Geometry: final body of the model. Coordinates: model frame, mm. A direction names the side the tool comes from. Give positions to 0.01 mm unless a question says otherwise; leave off trailing zeros. Write each loop counter-clockwise with the first axis right and the second up, starting at its lowest first coordinate (ties: lowest second). Pieces come first, ordered by that corner, then holes.
```python
from build123d import *

# Parameters (mm, degrees)
F1_DEPTH = 5
F2_R     = 1.669174
F2_R_2   = 1.66634
F3_DEPTH = 40.001
F4_R     = 1.5
F5_DEPTH = 4.001


with BuildPart() as f1:
    # F0 (on Right) → F1 (new body)
    with BuildSketch(Plane.YZ):
        Polygon((16, -8.883437), (0, -8.883437), (-16, -8.883437), (-16, 29.116563), (-20, 29.116563), (-20, -12.883437), (0, -12.883437), (20, -12.883437), (20, 29.116563), (16, 29.116563), align=None)
    extrude(amount=F1_DEPTH)

    # F2 (on face) → F3 (cut, through all)
    with BuildSketch(Plane.XZ.offset(20)):
        with Locations((2.5, 17.616563)):
            Circle(F2_R)
        with Locations((2.5, 2.616563)):
            Circle(F2_R_2)
    extrude(amount=-F3_DEPTH, mode=Mode.SUBTRACT)

    # F4 (on face) → F5 (cut, through all)
    with BuildSketch(Plane.XY.offset(-8.883437)):
        with Locations((2.5, -8)):
            Circle(F4_R)
        with Locations((2.5, 8)):
            Circle(F4_R)
    extrude(amount=-F5_DEPTH, mode=Mode.SUBTRACT)


solid = f1.part
```
Item 1: Section D-D, the plane z = 17. Return the cut outline in (x, y), plus the area to 3 significant figures.
Found:
outline: (0, -20) - (0.95, -20) - (0.95, -16) - (0, -16) - close; (0, 16) - (0.95, 16) - (0.95, 20) - (0, 20) - close; (4.05, -20) - (5, -20) - (5, -16) - (4.05, -16) - close; (4.05, 16) - (5, 16) - (5, 20) - (4.05, 20) - close
area: 15.2 mm2
Item 2: Pull-direction query (X, two-part tool) for faces 1 (the face through (0, 1, -10)), 2 (the face through (2, 0, -8.883)), 3 (the face through (5, 1, -10)), 4 (the face through (0.832, -18.028, 17.69)); classes: +X half, -X half, draft (parallel to the pull), parting line (faces both ways), or undercut.
Found:
face 1: -X half
face 2: draft
face 3: +X half
face 4: undercut
Item 3: Section C-C, the plane z = -4.5. Return the cut outline in (x, y).
Found:
outline: (0, -20) - (5, -20) - (5, -16) - (0, -16) - close; (0, 16) - (5, 16) - (5, 20) - (0, 20) - close
Item 4: Section B-B, the plane x = 2.5. State how many separate pieces and enclosed holes the cut face has, plus the area to 3 significant figures.
Found:
separate pieces: 7
enclosed holes: 0
area: 387 mm2
Item 5: Line query: L1, parallel to Z at x = 2.5, y = 17.4; L2, parallel to Y at x = 2.5, z = -12.05; L3, parallel to Y at x = 3.75, z = -7. Output: solid intervals per line, ascending.
Found:
L1: z = -12.88 to 0.95, 4.28 to 15.95, 19.29 to 29.12
L2: y = -20 to -9.5, -6.5 to 6.5, 9.5 to 20
L3: y = -20 to -16, 16 to 20
Item 6: Section A-A, the plane y = 8. Return the cut outline in (x, z), plus the area to 3 significant figures.
Found:
outline: (0, -12.88) - (1, -12.88) - (1, -8.88) - (0, -8.88) - close; (4, -12.88) - (5, -12.88) - (5, -8.88) - (4, -8.88) - close
area: 8.00 mm2
Item 7: Reachability of faces 5 (the face through (0.832, 17.972, 17.69)), 6 (the face through (2, 16, 10)) from +Z, -Z, +X, -X, +Y, -Y: full face, straight path, thin tool, end or side. Return the list, or none.
Found:
face 5: +Y, -Y
face 6: +Z, +X, -X
Item 8: Pin query (flat end, axial travel): pin 1 Ø1.5 at (x, y) = (2, 12.5) entering from +Z. Return the tip coordinate at first contact, or that it passes through.
Found:
pin 1: stops at z = -8.88
